Autodesk Inventor part; units mm, degrees
ref_plane "Start Plane" through (0, 0, 5) normal (0, 0, 1) x (1, 0, 0)
ref_plane "End Plane" through (0, 0, 69.5885) normal (0, 0, 1) x (1, 0, 0)
ref_plane "Work Plane4" through (7, 153.7024, 120.5399) normal (0, -0.3241, 0.946) x (1, 0, 0)
ref_plane "Start Plane" through (0, 0, 5) normal (0, 0, 1) x (1, 0, 0)
ref_plane "End Plane" through (0, 0, 69.5885) normal (0, 0, 1) x (1, 0, 0)
sketch "Sketch" plane through (0, 0, 0) normal (0, 0, 1) x (1, 0, 0)
  line L0 (5, -5) -> (-5, -5)
  line L1 (-5, -5) -> (-5, 5)
  line L2 (-5, 5) -> (5, 5)
  line L3 (5, 5) -> (5, -5)
  line L4 (-6, 0) -> (8, 0) construction
  line L5 (0, -30) -> (0, 40) construction
  line L6 (0, 54) -> (0, -44) construction
  line L7 (-9.2, 0) -> (13.2, 0) construction
  dimension "d0" = 10
  dimension "d1" = 10
  dimension "d4" = 5
  dimension "d5" = 5
extrude "Body" add sketch "Sketch" along normal up to surface (64.5885 mm away) from surface at 5
sketch "Sketch3" plane through (0, 0, 0) normal (0, 0, 1) x (1, 0, 0)
  line L0 (0, 0) -> (10, 0)
ref_plane "Work Plane3" through (0, 0, 0) normal (0, -1, 0) x (1, 0, 0)
sketch "Sketch4" plane through (0, 0, 0) normal (0, -1, 0) x (1, 0, 0)
  line L0 (-2, 5) -> (12, 5)
  line L1 (-2, 69.5885) -> (12, 69.5885)
  dimension "d9" = 64.5885
ref_plane "Work Plane4" through (7, 153.7024, 120.5399) normal (0, -0.3241, 0.946) x (1, 0, 0)
split "Split1" plane through (7, 153.7024, 120.5399) removes the side toward (0, -0.3241, 0.946)
ref_plane "Work Plane15" through (10.0028, -61.5702, 5) normal (0, 0, -1) x (-1, 0, 0)
split "Split12" plane through (10.0028, -61.5702, 5) removes the side toward (0, 0, -1)
equation "\"d0\" = G_W"
equation "\"d1\" = G_H"
equation "\"d4\" = 0.5 * d1"
equation "\"d5\" = 0.5 * d0"
equation "\"d2\" = G_L"
equation "\"G_W\" = 10"
equation "\"G_H\" = 10"
equation "\"G_L\" = d9"
equation "\"G_OFFSET_START\" = -5"
equation "\"G_OFFSET_END\" = -8.85593"
equation "\"d6\" = -G_OFFSET_START"
equation "\"d7\" = G_OFFSET_END + B_L"
equation "\"B_L\" = 78.44444"
properties part number "ISO 1035/2 - 10 x 10 - 64,59" material "Steel, Mild"
Here's how the part is built. I have some questions about the finished solid (model axes, mm). Round coordinates to 2 decimals unless told otherwise and drop trailing zeros. Loops run counter-clockwise (first coordinate to the right, second up) from the corner with the lowest first, then second, coordinate; pieces in that order, holes last. Notation, with made-up numbers: (78.5, 83) -> (99.5, 83) arc R21 cw to (99.5, 89) -> close; hole circle Ø8 at (42, 12.5). An arc over 180 degrees is marked (long way). Write each question's results on one line, items separated by ' | '.
(1) For P1, Ø5, axis at x = 2.5, y = -3, coming from the +Z side; P2, Ø1.5, axis at x = 2.5, y = -1, coming from the +Z side, each with a flat end and sliding along its axis, tell me the tip position at first contact or that it passes through.
Worked answers:
P1: z = 67.71 | P2: z = 67.8
(2) If we section it at B-B, the plane y = -4: List the corners of the cut face in (x, z) for me.
Worked answers:
outline: (-5, 5) -> (5, 5) -> (5, 66.51) -> (-5, 66.51) -> close
(3) If I drill on L1, parallel to Z at x = 1, y = -1.5; L2, parallel to Z at x = 3, y = 0, over which ranges is the centre line in solid material (lowest first)?
Worked answers:
L1: 5 to 67.37 | L2: 5 to 67.88
(4) If we section it at C-C, the plane y = 1.25: List the corners of the cut face in (x, z) for me, then the cut area to 3 significant figures.
Worked answers:
outline: (-5, 5) -> (5, 5) -> (5, 68.31) -> (-5, 68.31) -> close | area: 633 mm2
